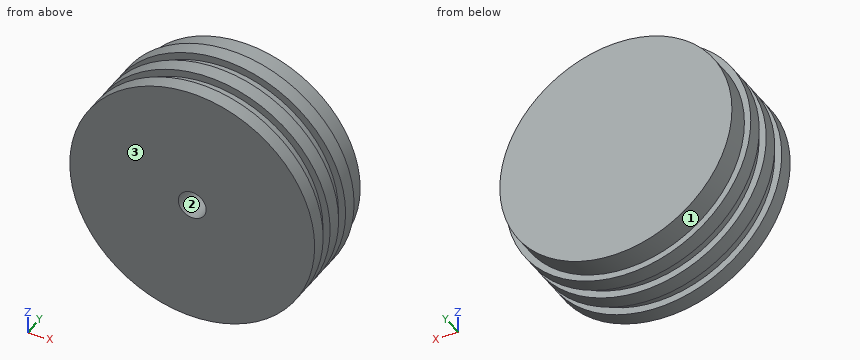
```python
from build123d import *

# Parameters (mm, degrees)
TAP_DRILL_FOR_3_8_16_TAP1_D     = 7.9375
TAP_DRILL_FOR_3_8_16_TAP1_DEPTH = 15.875
TAP_DRILL_FOR_3_8_16_TAP1_TIP   = 2.384665582


with BuildPart() as part:
    # Sketch8 → Revolve1 (revolve)
    with BuildSketch(Plane.XY):
        Polygon((0, 0), (0, 26.416), (-33.0835, 26.416), (-33.0835, 20.066), (-34.8996, 20.066), (-34.8996, 15.748), (-32.8676, 15.748), (-32.8676, 12.192), (-34.8996, 12.192), (-34.8996, 7.874), (-32.8676, 7.874), (-32.8676, 4.318), (-34.8996, 4.318), (-34.8996, 0), align=None)
    revolve(axis=Axis((0, 0, 0), (0, 1, 0)))

    # Tap Drill for 3/8-16 Tap1
    with Locations(Plane(origin=(0, 0, 0), x_dir=(-1, 0, 0), z_dir=(0, -1, 0))):
        with Locations((0, 0)):
            Hole(TAP_DRILL_FOR_3_8_16_TAP1_D / 2, depth=TAP_DRILL_FOR_3_8_16_TAP1_DEPTH)
            with Locations((0, 0, -(TAP_DRILL_FOR_3_8_16_TAP1_DEPTH + TAP_DRILL_FOR_3_8_16_TAP1_TIP / 2))):  # 118° drill point
                Cone(0, TAP_DRILL_FOR_3_8_16_TAP1_D / 2, TAP_DRILL_FOR_3_8_16_TAP1_TIP, mode=Mode.SUBTRACT)


solid = part.part
```
Geometry check sheet. Reference: the model listing, model coordinates, mm. Face numbers are marked on the shaded views. Give positions to 0.01 mm unless a question says otherwise; leave off trailing zeros. Loops run counter-clockwise (first coordinate to the right, second up) from the corner with the lowest first, then second, coordinate; pieces in that order, holes last. Notation, with made-up numbers: M 67,-12 L 125,-12 A15 ccw 125,13 Z; hole C 29,24.25 d2. An arc over 180 degrees is marked long. Answer as CSV lines item,"result".
Item 1: Cross-section at C-C on x = -7. Record the cut outline in (y, z), and give its area (3 significant figures).
Values:
outline,"M 0,-34.19 L 4.32,-34.19 L 4.32,-32.11 L 7.87,-32.11 L 7.87,-34.19 L 12.19,-34.19 L 12.19,-32.11 L 15.75,-32.11 L 15.75,-34.19 L 20.07,-34.19 L 20.07,-32.33 L 26.42,-32.33 L 26.42,32.33 L 20.07,32.33 L 20.07,34.19 L 15.75,34.19 L 15.75,32.11 L 12.19,32.11 L 12.19,34.19 L 7.87,34.19 L 7.87,32.11 L 4.32,32.11 L 4.32,34.19 L 0,34.19 Z"
area,"1,750 mm²"
Item 2: Material ranges on line 1 (Z direction, x = 0, y = 11); line 2 (X direction, y = 23.25, z = 12); line 3 (X direction, y = 6, z = 12.5), recorded low to high.
Values:
line 1,"z = -34.9 to -3.97, 3.97 to 34.9"
line 2,"x = -30.83 to 30.83"
line 3,"x = -30.4 to 30.4"
Item 3: Depth check by flat-ended pin: P1, Ø8, axis at x = -24, y = 21, coming from the +Z side; P2, Ø12, axis at x = 9.5, y = 12, coming from the -Z side; P3, Ø10, axis at x = 13, y = 11.5, coming from the +Z side. Enter the tip coordinate at first touch or a pass-through.
Values:
P1,"stops at z = 28.52"
P2,"stops at z = -34.72"
P3,"stops at z = 33.97"
Item 4: Cross-section at D-D on y = 6. Record the cut outline in (x, z), and give its area (3 significant figures).
Values:
outline,"C 0,0 d65.74; hole C 0,0 d7.94"
area,"3,340 mm²"
Item 5: Cross-section at B-B on z = -18.5. Record the cut outline in (x, y), and give its area (3 significant figures).
Values:
outline,"M -29.59,0 L 29.59,0 L 29.59,4.32 L 27.17,4.32 L 27.17,7.87 L 29.59,7.87 L 29.59,12.19 L 27.17,12.19 L 27.17,15.75 L 29.59,15.75 L 29.59,20.07 L 27.43,20.07 L 27.43,26.42 L -27.43,26.42 L -27.43,20.07 L -29.59,20.07 L -29.59,15.75 L -27.17,15.75 L -27.17,12.19 L -29.59,12.19 L -29.59,7.87 L -27.17,7.87 L -27.17,4.32 L -29.59,4.32 Z"
area,"1,500 mm²"
Item 6: Cross-section at A-A on y = 2.25. Record the cut outline in (x, z), and give its area (3 significant figures).
Values:
outline,"C 0,0 d69.8; hole C 0,0 d7.94"
area,"3,780 mm²"
Item 7: Release check for a two-part mould opening along X. For the marked faces 1, 2 and 3 record: pulls with the +X half, pulls with the -X half, needs draft (parallel to the pull), parting line crosses it, or undercut.
Values:
face 1,"parting line crosses it"
face 2,"undercut"
face 3,"needs draft"
